Here's how the part is built. I have some questions about the finished solid (model axes, mm). A direction names the side the tool comes from. Round coordinates to 2 decimals unless told otherwise and drop trailing zeros. Write each loop counter-clockwise with the first axis right and the second up, starting at its lowest first coordinate (ties: lowest second). Pieces come first, ordered by that corner, then holes. Notation, with made-up numbers: M -13.75,54.5 L 27.25,54.5 A18 ccw 27.25,82.5 Z; hole C 66.5,64 d8. An arc over 180 degrees is marked long. Use a Markdown table: item, result. Add a question column.
```python
from build123d import *

# Parameters (mm, degrees)
SKETCH1_R           = 1.5
SKETCH1_W           = 10
SKETCH1_H           = 3
BOSS_EXTRUDE1_DEPTH = 3


with BuildPart() as part:
    # Sketch1 → Boss-Extrude1 (new body)
    with BuildSketch(Plane(origin=(0, 0, 0), x_dir=(1, 0, 0), z_dir=(0, 1, 0))):
        Polygon((-26, -30), (-26, -60), (26, -60), (26, -30), (29, -30), (29, -20), (26, -20), (26, 20), (29, 20), (29, 30), (26, 30), (26, 60), (-26, 60), (-26, 30), (-29, 30), (-29, 20), (-26, 20), (-26, -20), (-29, -20), (-29, -30), align=None)
        with Locations((22.6, -52.6)):
            Circle(SKETCH1_R, mode=Mode.SUBTRACT)
        with Locations((-13.6, 7)):
            Circle(SKETCH1_R, mode=Mode.SUBTRACT)
        with Locations((0, -57.5)):
            Rectangle(SKETCH1_W, SKETCH1_H, mode=Mode.SUBTRACT)
        with Locations((0, 57.5)):
            Rectangle(SKETCH1_W, SKETCH1_H, mode=Mode.SUBTRACT)
    extrude(amount=BOSS_EXTRUDE1_DEPTH)


solid = part.part
```
Item 1: Imagine slicing it at C-C on y = 0.5. Count the separate pieces of the cut face and the enclosed holes in it, plus the area to 3 significant figures.
Item 2: For pin 1 Ø0.9 at (y, z) = (1, -38.5) entering from -X; pin 2 Ø0.9 at (x, y) = (-27, 1) entering from +Z; pin 3 Ø1.5 at (x, y) = (-27.5, 1) entering from -Z, each with a flat end and sliding along its axis, tell me the tip position at first contact or that it passes through.
Item 3: Imagine slicing it at D-D on z = -40. List the corners of the cut face in (x, y) for me, plus the area to 3 significant figures.
Item 4: Imagine slicing it at B-B on x = -13.6. List the corners of the cut face in (y, z) for me.
Item 5: I need wall thicknesses on probe 1 along Z at (x, y) = (-13.6, 0.85); probe 2 along Z at (x, y) = (0.5, 1.2); probe 3 along X at (y, z) = (2.2, -7). Which ranges of each line are inside material? Lowest first, please. Write a range as from..to.
Item 6: If we mould it in two halves opening along Z, with no side actions, what happens to faces 1 (the face through (28, 1, -30)), 2 (the face through (29, 1, 25)), 3 (the face through (26, 1, 0))? For each: +Z half, -Z half, draft (parallel to the pull), parting line (faces both ways), or undercut.
Item 7: Imagine slicing it at A-A on z = -7. List the corners of the cut face in (x, y) for me, plus the area to 3 significant figures.
Item 8: On a 3-axis mill with a long thin cutter (end or side, diameter ignored), from which of +Z, -Z, +X, -X, +Y, -Y can I reach the whole of each face in a straight line? I mean faces 4 (the face through (0, 1, -59)), 5 (the face through (-27, 1, -30)), 6 (the face through (-28, 1, 30)), 7 (the face through (27, 1, 30)). Say none if no direction works.
The answers:
| question | item | result |
|---|---|---|
| 1 | separate pieces | 1 |
| 1 | enclosed holes | 4 |
| 1 | area | 6,290 mm² |
| 2 | pin 1 | x = -26 |
| 2 | pin 2 | z = 30 |
| 2 | pin 3 | z = -30 |
| 3 | outline | M -26,0 L 26,0 L 26,3 L -26,3 Z |
| 3 | area | 156 mm² |
| 4 | outline | M 0,-60 L 3,-60 L 3,-8.5 L 0,-8.5 Z; M 0,-5.5 L 3,-5.5 L 3,60 L 0,60 Z |
| 5 | probe 1 | -60..-8.5, -5.5..60 |
| 5 | probe 2 | -60..-59, -56..56, 59..60 |
| 5 | probe 3 | -26..-15.1, -12.1..26 |
| 6 | face 1 | -Z half |
| 6 | face 2 | draft |
| 6 | face 3 | undercut |
| 7 | outline | M -26,0 L -15.1,0 L -15.1,3 L -26,3 Z; M -12.1,0 L 26,0 L 26,3 L -12.1,3 Z |
| 7 | area | 147 mm² |
| 8 | face 4 | +Y, -Y |
| 8 | face 5 | -Z, -X, +Y, -Y |
| 8 | face 6 | +Z, -X, +Y, -Y |
| 8 | face 7 | +Z, +X, +Y, -Y |
